from build123d import *

# Parameters (mm, degrees)
F1_DEPTH       = 76.2
F2_DEPTH       = 76.2
F4_D           = 15.24
F4_DEPTH       = 10.16
F4_CBORE_D     = 40.64
F4_CBORE_DEPTH = 10.16
F4_TIP         = 4.578557917
F5_R           = 10.16
F6_R           = 10.16
F8_DEPTH       = 27.94


with BuildPart() as f1:
    # F0 (on Right) → F1 (new body)
    with BuildSketch(Plane.YZ):
        Polygon((0, 35.56), (0, 0), (35.56, 0), (71.12, 35.56), (71.12, 71.12), (35.56, 71.12), align=None)
    extrude(amount=F1_DEPTH)

    # F2 (add): a face of the model
    f2_faces = [f1.faces().sort_by_distance(p)[0] for p in [
        (38.1, 0, 17.78),
    ]]
    extrude(f2_faces, amount=F2_DEPTH)

    # F4
    with Locations(Plane.XY.offset(35.56)):
        with Locations((38.1, -38.1)):
            CounterBoreHole(F4_D / 2, F4_CBORE_D / 2, F4_CBORE_DEPTH, depth=F4_DEPTH)
            with Locations((0, 0, -(F4_DEPTH + F4_TIP / 2))):  # 118° drill point
                Cone(0, F4_D / 2, F4_TIP, mode=Mode.SUBTRACT)

    # F5
    f5_edges = [f1.edges().sort_by_distance(p)[0] for p in [
        (76.2, -76.2, 17.78),
    ]]
    fillet(f5_edges, radius=F5_R)

    # F6
    f6_edges = [f1.edges().sort_by_distance(p)[0] for p in [
        (0, -76.2, 17.78),
    ]]
    fillet(f6_edges, radius=F6_R)

    # F7 (on face) → F8 (cut)
    with BuildSketch(Plane.XY.offset(71.12)):
        with BuildLine():
            Line((60.9591351744, 60.9599999509), (15.5202967077, 60.9548429896))
            ThreePointArc((15.5202967077, 60.9548429896), (7.6251627493, 53.6204525726), (14.9593915626, 45.7251684914))
            Line((14.9593915626, 45.7251684914), (15.5188972549, 45.7251056264))
            Line((15.5188972549, 45.7251056264), (60.9591438178, 45.7200000481))
            ThreePointArc((60.9591438178, 45.7200000481), (68.5799999863, 53.3400043217), (60.9591351744, 60.9599999509))
        make_face()
    extrude(amount=-F8_DEPTH, mode=Mode.SUBTRACT)


solid = f1.part
Model file for the job. Use its own axes, mm. A direction names the side the tool comes from. Give positions to 0.01 mm unless a question says otherwise; leave off trailing zeros. Order: outer loops, then holes, each group sorted by start corner. A loop starts at its lowest first (then second) coordinate and runs counter-clockwise, first axis right, second up. Notation, with made-up numbers: M 11.5,-38 L 47.5,-38 A22 cw 47.5,-30 Z; hole C 16.25,45 d7. An arc over 180 degrees is marked long. Write item = value, one per line.
Q1. Cut at C-C, the plane x = 21. List the corners of the cut face in (y, z).
Derived:
outline = M -76.2,0 L 35.56,0 L 71.12,35.56 L 71.12,71.12 L 60.96,71.12 L 60.96,43.18 L 45.72,43.18 L 45.72,71.12 L 35.56,71.12 L 0,35.56 L -27.12,35.56 L -27.12,25.4 L -49.08,25.4 L -49.08,35.56 L -76.2,35.56 Z
Q2. Two-plate mould, pull along Y, no slides. Class faces 4 (the cylindrical face through (7.633, 53.788, 57.346)), 5 (the flat face through (37.6, 61.5, 71.12)), 6 (the cylindrical face through (3.055, -73.303, 17.531)): pulls with the +Y half, pulls with the -Y half, needs draft (parallel to the pull), parting line crosses it, or undercut.
Derived:
face_4 = undercut
face_5 = needs draft
face_6 = pulls with the -Y half
Q3. Flat gauge pins, fed straight in: pin 1 (5 mm diameter, centred on x = 39, y = -4.5, fed in from -Z); pin 2 (4 mm diameter, centred on x = 62, z = 7.5, fed in from +Y); pin 3 (20.5 mm diameter, centred on x = 47, y = -43.5, fed in from +Z). Where does each tip first touch, or does it go through?
Derived:
pin_1 = 0
pin_2 = 45.06
pin_3 = 35.56
Q4. Tool access for faces 1 (the cylindrical face through (73.145, -73.303, 17.531)), 2 (the flat face through (47, -38, 25.4)), 3 (the flat face through (54, -54, 35.56)): list every direction of +Z, -Z, +X, -X, +Y, -Y with a clear straight run to the whole face (end or side of a thin tool).
Derived:
face_1 = +Z, -Z, +X, -Y
face_2 = +Z
face_3 = +Z, +X, -X, -Y
Q5. Cut at A-A, the plane z = 46. List the corners of the cut face in (x, y), then the cut area to 3 significant figures.
Derived:
outline = M 0,10.44 L 76.2,10.44 L 76.2,71.12 L 0,71.12 Z; hole M 14.96,45.73 L 60.96,45.72 A7.62 ccw 60.96,60.96 L 15.52,60.95 A7.62 ccw Z
area = 3,740 mm2
Q6. Cut at B-B, the plane y = 53.34. List the corners of the cut face in (x, z).
Derived:
outline = M 0,17.78 L 76.2,17.78 L 76.2,71.12 L 68.58,71.12 L 68.58,43.18 L 7.62,43.18 L 7.62,71.12 L 0,71.12 Z
Q7. Cut at D-D, the plane z = 62. List the corners of the cut face in (x, y), then the cut area to 3 significant figures.
Derived:
outline = M 0,26.44 L 76.2,26.44 L 76.2,71.12 L 0,71.12 Z; hole M 14.96,45.73 L 60.96,45.72 A7.62 ccw 60.96,60.96 L 15.52,60.95 A7.62 ccw Z
area = 2,530 mm2
Q8. Drill centre lines: line 1 (X direction, y = -38, z = 30); line 2 (Z direction, x = 45, y = -4); line 3 (Y direction, x = 53.5, z = 64.5). Where is each one in solid material? Low to high. Write a range as [from, to].
Derived:
line_1 = [0, 17.78], [58.42, 76.2]
line_2 = [0, 35.56]
line_3 = [28.94, 45.72], [60.96, 71.12]
